```python
from build123d import *

# Parameters (mm, degrees)
F0_R     = 1.5
F1_DEPTH = 2


with BuildPart() as f1:
    # F0 (on Top) → F1 (new body)
    with BuildSketch(Plane.XY):
        Polygon((-42.367958, -92), (-25, -95.822892), (25, -95.822892), (42.367958, -92), (25, -57.454384), (42.367958, -42), (25, -12.163068), (42.367958, 0), (25, 29.917361), (42.367958, 40), (25, 60.158143), (42.367958, 73.368201), (42.367958, 85.368201), (25, 104.778975), (-25, 104.778975), (-42.367958, 85.368201), (-42.367958, 73.368201), (-25, 60.158143), (-42.367958, 40), (-25, 29.917361), (-42.367958, 0), (-25, -12.163068), (-42.367958, -42), (-25, -57.454384), align=None)
        with Locations((-20, -88)):
            Circle(F0_R, mode=Mode.SUBTRACT)
        with Locations((-20, -68.25)):
            Circle(F0_R, mode=Mode.SUBTRACT)
        with Locations((0, -88)):
            Circle(F0_R, mode=Mode.SUBTRACT)
        with Locations((20, -88)):
            Circle(F0_R, mode=Mode.SUBTRACT)
        with Locations((20, -68.25)):
            Circle(F0_R, mode=Mode.SUBTRACT)
        with Locations((-32, 86)):
            Circle(F0_R, mode=Mode.SUBTRACT)
        with Locations((-20, 95)):
            Circle(F0_R, mode=Mode.SUBTRACT)
        with Locations((0, 95)):
            Circle(F0_R, mode=Mode.SUBTRACT)
        with Locations((20, 95)):
            Circle(F0_R, mode=Mode.SUBTRACT)
        with Locations((32, 86)):
            Circle(F0_R, mode=Mode.SUBTRACT)
    extrude(amount=F1_DEPTH)


solid = f1.part
```
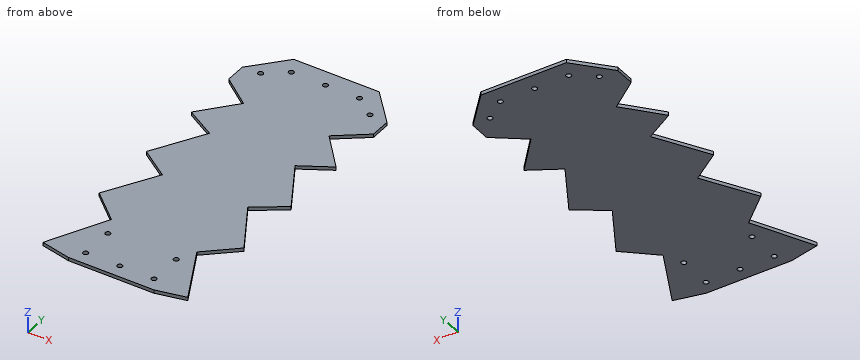
Can you work these out from the model? Positions are in its coordinate system, mm. Round coordinates to 2 decimals unless told otherwise and drop trailing zeros. Loops run counter-clockwise (first coordinate to the right, second up) from the corner with the lowest first, then second, coordinate; pieces in that order, holes last. Notation, with made-up numbers: (0, 45.25) -> (50, 45.25) arc R14 cw to (50, 49.25) -> close; hole circle Ø4 at (-36, -35). An arc over 180 degrees is marked (long way). One line per item, written item: value. Start each with the question number.
1. If we section it at B-B, the plane y = 27.5: Write out the boundary of the cut face in (x, z).
2. If we section it at A-A, the plane z = 0.85: Give the number of separate pieces and of enclosed holes in the cut face, then the cut area to 3 significant figures.
3. For pin 1 (1 mm diameter, centred on y = 31.5, z = 0, fed in from -X); pin 2 (1 mm diameter, centred on y = 20, z = 0.5, fed in from -X), each with a flat end and sliding along its axis, tell me the tip position at first contact or that it passes through.
4. If I drill on probe 1 along Y at (x, z) = (0, 1.55); probe 2 along Y at (x, z) = (37, 1); probe 3 along Y at (x, z) = (20, 0.7), over which ranges is the centre line in solid material (lowest first)?
Calculated:
1. outline: (-26.4, 0) -> (26.4, 0) -> (26.4, 2) -> (-26.4, 2) -> close
2. separate pieces: 1
2. enclosed holes: 10
2. area: 13,700 mm²
3. pin 1: stops at x = -28.59
3. pin 2: stops at x = -31.05
4. probe 1: y = -95.82 to -89.5, -86.5 to 93.5, 96.5 to 104.78
4. probe 2: y = -93.18 to -81.32, -46.78 to -32.78, -3.76 to 9.25, 36.88 to 46.23, 69.29 to 91.37
4. probe 3: y = -95.82 to -89.5, -86.5 to -69.75, -66.75 to 93.5, 96.5 to 104.78
